```python
from build123d import *

# Parameters (mm, degrees)
SKETCH1_R               = 2.5
BOSS_EXTRUDE1_DEPTH     = 50
SKETCH2_R               = 2
CUT_EXTRUDE1_DEPTH      = 1
CUT_EXTRUDE1_DEPTH_BACK = 21


with BuildPart() as part:
    # Sketch1 → Boss-Extrude1 (new body)
    with BuildSketch(Plane.XY):
        with BuildLine():
            Line((-9.707106781, -3.2), (-8.6, -3.2))
            Line((-8.6, -3.2), (-8.6, -7.185786438))
            Line((-8.6, -7.185786438), (-3.445719569, -2.031506006))
            ThreePointArc((-3.445719569, -2.031506006), (-4, 0), (-3.445719569, 2.031506006))
            Line((-3.445719569, 2.031506006), (-8.6, 7.185786438))
            Line((-8.6, 7.185786438), (-8.6, 3.2))
            Line((-8.6, 3.2), (-9.707106781, 3.2))
            Line((-9.707106781, 3.2), (-9.707106781, 3.877544562))
            Line((-9.707106781, 3.877544562), (-10, 3.877544562))
            Line((-10, 3.877544562), (-10, 9))
            ThreePointArc((-10, 9), (-9.707106781, 9.707106781), (-9, 10))
            Line((-9, 10), (-3.877544562, 10))
            Line((-3.877544562, 10), (-3.877544562, 9.707106781))
            Line((-3.877544562, 9.707106781), (-3.2, 9.707106781))
            Line((-3.2, 9.707106781), (-3.2, 8.6))
            Line((-3.2, 8.6), (-7.185786438, 8.6))
            Line((-7.185786438, 8.6), (-2.031506006, 3.445719569))
            ThreePointArc((-2.031506006, 3.445719569), (0, 4), (2.031506006, 3.445719569))
            Line((2.031506006, 3.445719569), (7.185786438, 8.6))
            Line((7.185786438, 8.6), (3.2, 8.6))
            Line((3.2, 8.6), (3.2, 9.707106781))
            Line((3.2, 9.707106781), (3.877544562, 9.707106781))
            Line((3.877544562, 9.707106781), (3.877544562, 10))
            Line((3.877544562, 10), (9, 10))
            ThreePointArc((9, 10), (9.707106781, 9.707106781), (10, 9))
            Line((10, 9), (10, 3.877544562))
            Line((10, 3.877544562), (9.707106781, 3.877544562))
            Line((9.707106781, 3.877544562), (9.707106781, 3.2))
            Line((9.707106781, 3.2), (8.6, 3.2))
            Line((8.6, 3.2), (8.6, 7.185786438))
            Line((8.6, 7.185786438), (3.445719569, 2.031506006))
            ThreePointArc((3.445719569, 2.031506006), (4, 0), (3.445719569, -2.031506006))
            Line((3.445719569, -2.031506006), (8.6, -7.185786438))
            Line((8.6, -7.185786438), (8.6, -3.2))
            Line((8.6, -3.2), (9.707106781, -3.2))
            Line((9.707106781, -3.2), (9.707106781, -3.877544562))
            Line((9.707106781, -3.877544562), (10, -3.877544562))
            Line((10, -3.877544562), (10, -9))
            ThreePointArc((10, -9), (9.707106781, -9.707106781), (9, -10))
            Line((9, -10), (3.877544562, -10))
            Line((3.877544562, -10), (3.877544562, -9.707106781))
            Line((3.877544562, -9.707106781), (3.2, -9.707106781))
            Line((3.2, -9.707106781), (3.2, -8.6))
            Line((3.2, -8.6), (7.185786438, -8.6))
            Line((7.185786438, -8.6), (2.031506006, -3.445719569))
            ThreePointArc((2.031506006, -3.445719569), (0, -4), (-2.031506006, -3.445719569))
            Line((-2.031506006, -3.445719569), (-7.185786438, -8.6))
            Line((-7.185786438, -8.6), (-3.2, -8.6))
            Line((-3.2, -8.6), (-3.2, -9.707106781))
            Line((-3.2, -9.707106781), (-3.877544562, -9.707106781))
            Line((-3.877544562, -9.707106781), (-3.877544562, -10))
            Line((-3.877544562, -10), (-9, -10))
            ThreePointArc((-9, -10), (-9.707106781, -9.707106781), (-10, -9))
            Line((-10, -9), (-10, -3.877544562))
            Line((-10, -3.877544562), (-9.707106781, -3.877544562))
            Line((-9.707106781, -3.877544562), (-9.707106781, -3.2))
        make_face()
        Circle(SKETCH1_R, mode=Mode.SUBTRACT)
    extrude(amount=BOSS_EXTRUDE1_DEPTH)

    # Sketch2 → Cut-Extrude1 (cut, two sides)
    with BuildSketch(Plane(origin=(0, 10, 0), x_dir=(1, 0, 0), z_dir=(0, 1, 0))) as cut_extrude1_sk:
        with Locations((0, -42)):
            Circle(SKETCH2_R)
    extrude(amount=CUT_EXTRUDE1_DEPTH, mode=Mode.SUBTRACT)
    extrude(cut_extrude1_sk.sketch, amount=-CUT_EXTRUDE1_DEPTH_BACK, mode=Mode.SUBTRACT)


solid = part.part
```
Verification items for the finished model (mm, model axes). A direction names the side the tool comes from. Give positions to 0.01 mm unless a question says otherwise; leave off trailing zeros. Order: outer loops, then holes, each group sorted by start corner. A loop starts at its lowest first (then second) coordinate and runs counter-clockwise, first axis right, second up. Notation, with made-up numbers: (-18.75, 44) -> (-1.75, 44) arc R29 ccw to (-1.75, 82) -> close; hole circle Ø3 at (-16.75, 89.25). An arc over 180 degrees is marked (long way). One line per item, written item: value.
(1) Sectioned sample at C-C on y = -6.5. Record the cut outline in (x, z), then the cut area to 3 significant figures.
Final values:
outline: (-10, 0) -> (-8.6, 0) -> (-8.6, 50) -> (-10, 50) -> close; (-7.91, 0) -> (-5.09, 0) -> (-5.09, 50) -> (-7.91, 50) -> close; (5.09, 0) -> (7.91, 0) -> (7.91, 50) -> (5.09, 50) -> close; (8.6, 0) -> (10, 0) -> (10, 50) -> (8.6, 50) -> close
area: 423 mm^2
(2) Sectioned sample at A-A on x = 0. Record the cut outline in (y, z).
Final values:
outline: (-4, 0) -> (-2.5, 0) -> (-2.5, 40) -> (-4, 40) -> close; (-4, 44) -> (-2.5, 44) -> (-2.5, 50) -> (-4, 50) -> close; (2.5, 0) -> (4, 0) -> (4, 40) -> (2.5, 40) -> close; (2.5, 44) -> (4, 44) -> (4, 50) -> (2.5, 50) -> close
(3) Sectioned sample at D-D on y = 8. Record the cut outline in (x, z).
Final values:
outline: (-10, 0) -> (-6.59, 0) -> (-6.59, 50) -> (-10, 50) -> close; (6.59, 0) -> (10, 0) -> (10, 50) -> (6.59, 50) -> close
(4) Sectioned sample at B-B on y = 0. Record the cut outline in (x, z), then the cut area to 3 significant figures.
Final values:
outline: (-4, 0) -> (-2.5, 0) -> (-2.5, 50) -> (-4, 50) -> close; (2.5, 0) -> (4, 0) -> (4, 50) -> (2.5, 50) -> close
area: 150 mm^2
(5) Gauge pin test, flat ends, axial feed: pin 1 (3 mm diameter, centred on y = -2, z = 20.5, fed in from +X); pin 2 (3 mm diameter, centred on x = 0, z = 42, fed in from +Y). Record the tip position at first contact, or that the pin passes through.
Final values:
pin 1: x = 9.71
pin 2: through
(6) Draft check along Y on faces 1 (the face through (-6, 10, 25)), 2 (the face through (-6.059, -4.645, 24.65)), 3 (the face through (6, -10, 25)). Enter one of: pulls with the +Y half, pulls with the -Y half, needs draft (parallel to the pull), parting line crosses it, or undercut.
Final values:
face 1: pulls with the +Y half
face 2: undercut
face 3: pulls with the -Y half
(7) Tool access check on faces 4 (the face through (-4, 0, 25)), 5 (the face through (5.987, -4.573, 24.65)), 6 (the face through (9, 3.2, 25)). Record the directions out of +Z, -Z, +X, -X, +Y, -Y that give a thin tool (end or side, any length) a straight path to the whole face; none if there is none.
Final values:
face 4: +Z, -Z, -X
face 5: +Z, -Z
face 6: +Z, -Z, +X
(8) Scan lines: line 1 along X through (y, z) = (-4.5, 45); line 2 along X through (y, z) = (-5, 36.5); line 3 along Y through (x, z) = (5.5, 20). Record each from-to range of solid material in increasing order. Write a range as [from, to].
Final values:
line 1: [-10, -8.6], [-5.91, -3.09], [3.09, 5.91], [8.6, 10]
line 2: [-10, -8.6], [-6.41, -3.59], [3.59, 6.41], [8.6, 10]
line 3: [-10, -8.6], [-6.91, -4.09], [4.09, 6.91], [8.6, 10]
